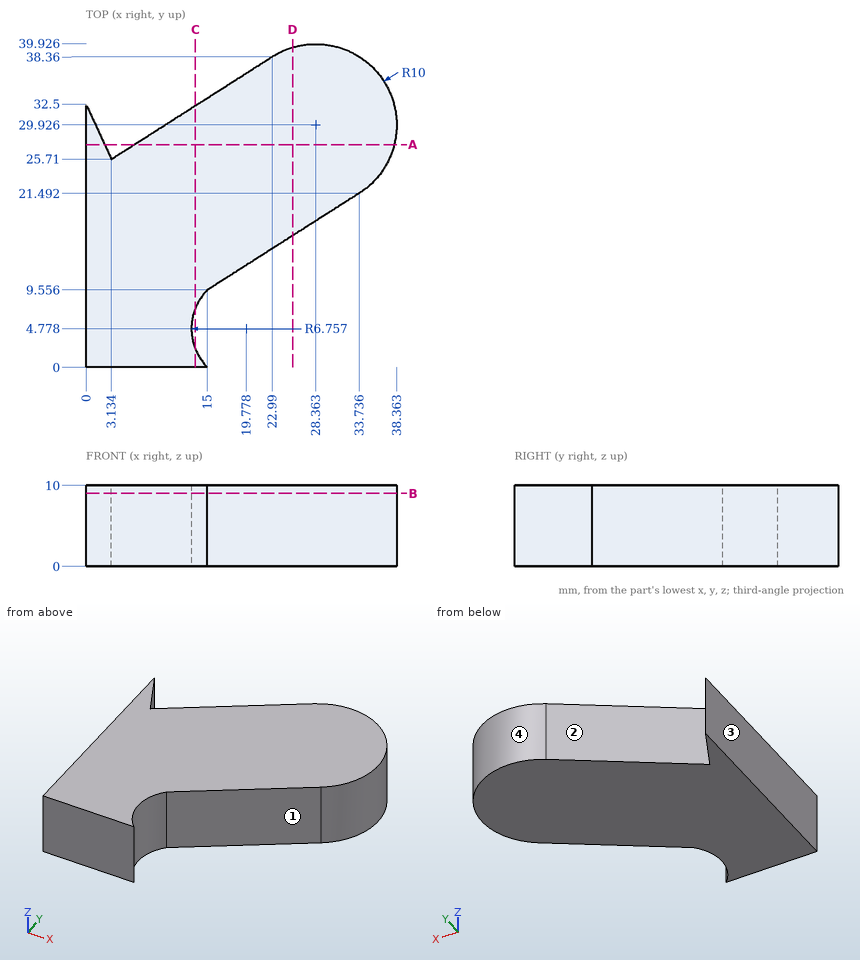
Here's the drawing with two shaded views (mm, measured from the low corner). I have some questions. Coordinates: 2 decimals unless noted, no trailing zeros. Write each loop counter-clockwise with the first axis right and the second up, starting at its lowest first coordinate (ties: lowest second). Pieces come first, ordered by that corner, then holes. Notation, with made-up numbers: (13.5, 79.5) -> (38.5, 79.5) arc R34 cw to (38.5, 114.5) -> close; hole circle Ø7 at (-19.75, -29). An arc over 180 degrees is marked (long way). Answer as CSV lines item,"result".
1) If we section it at A-A on y = 27.5: Please give me the cut outline in (x, z).
Check result:
outline,"(0, 0) -> (2.31, 0) -> (2.31, 10) -> (0, 10) -> close; (5.94, 0) -> (38.06, 0) -> (38.06, 10) -> (5.94, 10) -> close"
2) If we section it at D-D on x = 25.5: Please give me the cut outline in (y, z) (1 decimal).
Check result:
outline,"(16.2, 0) -> (39.5, 0) -> (39.5, 10) -> (16.2, 10) -> close"
3) If we mould it in two halves opening along X, with no side actions, what happens to the marked faces 1, 2, 3 and 4? For each: +X half, -X half, draft (parallel to the pull), parting line (faces both ways), or undercut.
Check result:
face 1,"+X half"
face 2,"undercut"
face 3,"-X half"
face 4,"parting line"
4) If we section it at C-C on x = 13.5: Please give me the cut outline in (y, z).
Check result:
outline,"(0, 0) -> (2.28, 0) -> (2.28, 10) -> (0, 10) -> close; (7.28, 0) -> (32.31, 0) -> (32.31, 10) -> (7.28, 10) -> close"
5) Will these pins go through, and if not, where does the flat tip stop? P1, Ø6, axis at x = 30.5, y = 15, coming from the +Z side; P2, Ø12, axis at x = 15.5, y = 12.5, coming from the -Z side; P3, Ø1.5, axis at y = 27.5, z = 5.5, coming from the +X side; P4, Ø6, axis at y = 12, z = 4, coming from the +X side (1 decimal).
Check result:
P1,"through"
P2,"z = 0"
P3,"x = 38.22"
P4,"x = 23.5"
6) If I drill on line 1 (X direction, y = 27, z = 2.25) (1 decimal); line 2 (X direction, y = 4.5, z = 7); line 3 (X direction, y = 31, z = 5.5) (1 decimal), over which ranges is the centre line in solid material (lowest first)? Write a range as from..to.
Check result:
line 1,"0..2.5, 5.2..37.9"
line 2,"0..13.03"
line 3,"0..0.7, 11.4..38.3"
7) If we section it at B-B on z = 9: Please give me the cut outline in (x, y) (1 decimal).
Check result:
outline,"(0, 0) -> (15, 0) arc R6.8 cw to (15, 9.6) -> (33.7, 21.5) arc R10 ccw to (23, 38.4) -> (3.1, 25.7) -> (0, 32.5) -> close"
